from build123d import *

# Parameters (mm, degrees)
BOX021_W                     = 4.2
BOX021_H                     = 6
BOX021_DEPTH                 = 15
BOX020_W                     = 4.2
BOX020_H                     = 6
BOX020_DEPTH                 = 15
BOX019_W                     = 4.2
BOX019_H                     = 6
BOX019_DEPTH                 = 15
BOX018_W                     = 4.2
BOX018_H                     = 6
BOX018_DEPTH                 = 15
BOX017_W                     = 10
BOX017_H                     = 10
BOX017_DEPTH                 = 32.4
PAD_DEPTH                    = 3
POCKET_DEPTH                 = 472.173047
POCKET_LINEARPATTERN_2_DEPTH = 472.173047
POCKET_LINEARPATTERN_3_DEPTH = 472.173047
POCKET_LINEARPATTERN_4_DEPTH = 472.173047
LINEARPATTERN001_COUNT       = 2
LINEARPATTERN001_PITCH       = 48.025


with BuildPart() as obj1:
    # Box021 → Box021 (new body)
    with BuildSketch(Plane(origin=(211.4, 8, 15.25), x_dir=(1, 0, 0), z_dir=(0, 0, 1))):
        with Locations((2.1, 3)):
            Rectangle(BOX021_W, BOX021_H)
    extrude(amount=BOX021_DEPTH)


with BuildPart() as obj2:
    # Box020 → Box020 (new body)
    with BuildSketch(Plane(origin=(8.4, 8, 15.25), x_dir=(1, 0, 0), z_dir=(0, 0, 1))):
        with Locations((2.1, 3)):
            Rectangle(BOX020_W, BOX020_H)
    extrude(amount=BOX020_DEPTH)


with BuildPart() as obj3:
    # Box019 → Box019 (new body)
    with BuildSketch(Plane(origin=(8.4, 8, 71.75), x_dir=(1, 0, 0), z_dir=(0, 0, 1))):
        with Locations((2.1, 3)):
            Rectangle(BOX019_W, BOX019_H)
    extrude(amount=BOX019_DEPTH)


with BuildPart() as obj4:
    # Box018 → Box018 (new body)
    with BuildSketch(Plane(origin=(211.4, 8, 71.75), x_dir=(1, 0, 0), z_dir=(0, 0, 1))):
        with Locations((2.1, 3)):
            Rectangle(BOX018_W, BOX018_H)
    extrude(amount=BOX018_DEPTH)


with BuildPart() as usbopening:
    # Box017 → Box017 (new body)
    with BuildSketch(Plane(origin=(211.5, 4.5, 36.3), x_dir=(1, 0, 0), z_dir=(0, 0, 1))):
        with Locations((5, 5)):
            Rectangle(BOX017_W, BOX017_H)
    extrude(amount=BOX017_DEPTH)


with BuildPart() as pocketed_back:
    # Sketch005 → Pad (new body)
    with BuildSketch(Plane.XZ):
        with BuildLine():
            Line((-99, 48.025), (99, 48.025))
            ThreePointArc((107, 40.025), (104.656854, 45.681854), (99, 48.025))
            Line((107, 40.025), (107, -40.025))
            ThreePointArc((99, -48.025), (104.656854, -45.681854), (107, -40.025))
            Line((99, -48.025), (-99, -48.025))
            ThreePointArc((-107, -40.025), (-104.656854, -45.681854), (-99, -48.025))
            Line((-107, -40.025), (-107, 40.025))
            ThreePointArc((-99, 48.025), (-104.656854, 45.681854), (-107, 40.025))
        make_face()
    extrude(amount=PAD_DEPTH)

    # Sketch006 (on Face10 of Pad) → Pocket (cut, through all)
    with BuildSketch(Plane.XZ.offset(3)):
        Polygon((-91, 38.769859), (-91, 9.255141), (-76.242641, 24.0125), align=None)
        Polygon((-86.757359, 43.0125), (-57.242641, 43.0125), (-72, 28.255141), align=None)
        Polygon((-67.757359, 24.0125), (-53, 38.769859), (-53, 9.255141), align=None)
        Polygon((-72, 19.769859), (-57.242641, 5.0125), (-86.757359, 5.0125), align=None)
    pocket = extrude(amount=-POCKET_DEPTH, mode=Mode.SUBTRACT)

    # Sketch006 LinearPattern 2 → Pocket LinearPattern 2 (cut, through all)
    with BuildSketch(Plane(origin=(48, -3, 0), x_dir=(1, 0, 0), z_dir=(0, -1, 0))):
        Polygon((-91, 38.769859), (-91, 9.255141), (-76.242641, 24.0125), align=None)
        Polygon((-86.757359, 43.0125), (-57.242641, 43.0125), (-72, 28.255141), align=None)
        Polygon((-67.757359, 24.0125), (-53, 38.769859), (-53, 9.255141), align=None)
        Polygon((-72, 19.769859), (-57.242641, 5.0125), (-86.757359, 5.0125), align=None)
    pocket_linearpattern_2 = extrude(amount=-POCKET_LINEARPATTERN_2_DEPTH, mode=Mode.SUBTRACT)

    # Sketch006 LinearPattern 3 → Pocket LinearPattern 3 (cut, through all)
    with BuildSketch(Plane(origin=(96, -3, 0), x_dir=(1, 0, 0), z_dir=(0, -1, 0))):
        Polygon((-91, 38.769859), (-91, 9.255141), (-76.242641, 24.0125), align=None)
        Polygon((-86.757359, 43.0125), (-57.242641, 43.0125), (-72, 28.255141), align=None)
        Polygon((-67.757359, 24.0125), (-53, 38.769859), (-53, 9.255141), align=None)
        Polygon((-72, 19.769859), (-57.242641, 5.0125), (-86.757359, 5.0125), align=None)
    pocket_linearpattern_3 = extrude(amount=-POCKET_LINEARPATTERN_3_DEPTH, mode=Mode.SUBTRACT)

    # Sketch006 LinearPattern 4 → Pocket LinearPattern 4 (cut, through all)
    with BuildSketch(Plane(origin=(144, -3, 0), x_dir=(1, 0, 0), z_dir=(0, -1, 0))):
        Polygon((-91, 38.769859), (-91, 9.255141), (-76.242641, 24.0125), align=None)
        Polygon((-86.757359, 43.0125), (-57.242641, 43.0125), (-72, 28.255141), align=None)
        Polygon((-67.757359, 24.0125), (-53, 38.769859), (-53, 9.255141), align=None)
        Polygon((-72, 19.769859), (-57.242641, 5.0125), (-86.757359, 5.0125), align=None)
    pocket_linearpattern_4 = extrude(amount=-POCKET_LINEARPATTERN_4_DEPTH, mode=Mode.SUBTRACT)

    # LinearPattern001: Pocket, Pocket LinearPattern 2, Pocket LinearPattern 3, Pocket LinearPattern 4 ×2
    with Locations(*[(0, 0, -i * LINEARPATTERN001_PITCH) for i in range(1, LINEARPATTERN001_COUNT)]):
        add(pocket, mode=Mode.SUBTRACT)
        add(pocket_linearpattern_2, mode=Mode.SUBTRACT)
        add(pocket_linearpattern_3, mode=Mode.SUBTRACT)
        add(pocket_linearpattern_4, mode=Mode.SUBTRACT)


with BuildPart() as pocketed_back_1:
    # Body placement: moved
    add(pocketed_back.part.moved(Location((112, 12.5, 58.5))))

    # Cut010: cut USBOpening
    add(usbopening.part, mode=Mode.SUBTRACT)

    # Cut011: cut obj4
    add(obj4.part, mode=Mode.SUBTRACT)

    # Cut012: cut obj3
    add(obj3.part, mode=Mode.SUBTRACT)

    # Cut013: cut obj2
    add(obj2.part, mode=Mode.SUBTRACT)

    # Cut014: cut obj1
    add(obj1.part, mode=Mode.SUBTRACT)


solid = pocketed_back_1.part
Could you check a few things on this model? Use its own coordinates, in mm. Give positions to 0.01 mm unless a question says otherwise; leave off trailing zeros. Write each loop counter-clockwise with the first axis right and the second up, starting at its lowest first coordinate (ties: lowest second). Pieces come first, ordered by that corner, then holes. Notation, with made-up numbers: (89, 17) -> (124, 17) arc R27 cw to (124, 52) -> close; hole circle Ø10 at (61.25, 16.25). An arc over 180 degrees is marked (long way). Answer as a JSON object with one key per item and string values.
Q1. Please list where these lines run through material, in increasing order: L1, parallel to Z at x = 55, y = 11.3 (3 decimals); L2, parallel to Z at x = 118.5, y = 10.6 (3 decimals); L3, parallel to Z at x = 186, y = 10.45 (1 decimal).
Taken from the geometry:
{"L1": "z = 10.475 to 23.73, 45.245 to 71.755, 93.27 to 106.525", "L2": "z = 10.475 to 21.23, 47.745 to 69.255, 95.77 to 106.525", "L3": "z = 10.5 to 15.5, 28.2 to 40.7, 53.5 to 63.5, 76.3 to 88.8, 101.5 to 106.5"}
Q2. We'd pull the mould along Z, two halves only. Please class faces 1 (the flat face through (113, 12.5, 59)), 2 (the flat face through (124.28, 10.98, 27.01)): released by +Z, released by -Z, zero draft, split by the parting line, or undercut.
Taken from the geometry:
{"face 1": "zero draft", "face 2": "undercut"}
Q3. Suppose I cut it at B-B on y = 10.95. Count the separate pieces of the cut face and the enclosed holes in it, then the cut area to 3 significant figures.
Taken from the geometry:
{"separate pieces": "1", "enclosed holes": "36", "area": "13,000 mm²"}
Q4. Will this pin go through, and if not, where does the flat tip stop? pin 1 Ø0.9 at (y, z) = (11, 39) entering from +X.
Taken from the geometry:
{"pin 1": "stops at x = 211.5"}
Q5. Suppose I cut it at A-A on x = 81. Write out the boundary of the cut face in (y, z) (1 decimal), then the cut area to 3 significant figures.
Taken from the geometry:
{"outline": "(9.5, 10.5) -> (12.5, 10.5) -> (12.5, 15.5) -> (9.5, 15.5) -> close; (9.5, 23.2) -> (12.5, 23.2) -> (12.5, 31.7) -> (9.5, 31.7) -> close; (9.5, 37.2) -> (12.5, 37.2) -> (12.5, 45.7) -> (9.5, 45.7) -> close; (9.5, 53.5) -> (12.5, 53.5) -> (12.5, 63.5) -> (9.5, 63.5) -> close; (9.5, 71.3) -> (12.5, 71.3) -> (12.5, 79.8) -> (9.5, 79.8) -> close; (9.5, 85.3) -> (12.5, 85.3) -> (12.5, 93.8) -> (9.5, 93.8) -> close; (9.5, 101.5) -> (12.5, 101.5) -> (12.5, 106.5) -> (9.5, 106.5) -> close", "area": "162 mm²"}
